Verification items for the finished model (mm, model axes). Face numbers are marked on the shaded views. A direction names the side the tool comes from. Give positions to 0.01 mm unless a question says otherwise; leave off trailing zeros. Loops run counter-clockwise (first coordinate to the right, second up) from the corner with the lowest first, then second, coordinate; pieces in that order, holes last. Notation, with made-up numbers: M -7.5,73.5 L 42.5,73.5 A25 ccw 42.5,89.5 Z; hole C 12.5,-35 d6. An arc over 180 degrees is marked long. Use CSV: the item, a comma, the result in double quotes.
from build123d import *

# Parameters (mm, degrees)
SKETCH1_W                 = 150
SKETCH1_H                 = 54.5
BOSS_EXTRUDE1_DEPTH       = 5
SKETCH2_W                 = 5
SKETCH2_H                 = 54.5
BOSS_EXTRUDE2_DEPTH       = 8
F_8_CLEARANCE_HOLE1_D     = 4.4958
F_8_CLEARANCE_HOLE1_DEPTH = 17
F_8_CLEARANCE_HOLE1_TIP   = 1.350674586
SKETCH7_W                 = 5
SKETCH7_H                 = 54.5
BOSS_EXTRUDE3_DEPTH       = 43
SKETCH8_R                 = 4.25
CUT_EXTRUDE1_DEPTH        = 4
RIB1_REACH                = 120.085
SKETCH10_WALL_W           = 279.571445908
SKETCH10_WALL_H           = 10
RIB3_REACH                = 120.085
SKETCH12_WALL_W           = 279.571445908
SKETCH12_WALL_H           = 10
SKETCH13_W                = 8
SKETCH13_H                = 2
BOSS_EXTRUDE4_DEPTH       = 5
SKETCH14_R                = 2
CUT_EXTRUDE2_DEPTH        = 2
SKETCH15_R                = 3.5
CUT_EXTRUDE3_DEPTH        = 1
F_8_CLEARANCE_HOLE2_D     = 4.4958
F_8_CLEARANCE_HOLE2_DEPTH = 17
F_8_CLEARANCE_HOLE2_TIP   = 1.350674586
SKETCH16_W                = 10
SKETCH16_H                = 12
BOSS_EXTRUDE5_DEPTH       = 20
SKETCH18_W                = 7
SKETCH18_H                = 7
CUT_EXTRUDE4_DEPTH        = 8


with BuildPart() as part:
    # Sketch1 → Boss-Extrude1 (new body)
    with BuildSketch(Plane(origin=(0, 0, 0), x_dir=(1, 0, 0), z_dir=(0, 1, 0))):
        with Locations((-18.112463826, -1.689393939)):
            Rectangle(SKETCH1_W, SKETCH1_H)
    extrude(amount=BOSS_EXTRUDE1_DEPTH)

    # Sketch2 → Boss-Extrude2 (add)
    with BuildSketch(Plane(origin=(0, 5, 0), x_dir=(1, 0, 0), z_dir=(0, 1, 0))):
        with Locations((-90.612463826, -1.689393939)):
            Rectangle(SKETCH2_W, SKETCH2_H)
    extrude(amount=BOSS_EXTRUDE2_DEPTH)

    # #8 Clearance Hole1
    with Locations(Plane(origin=(-93.112463826, 9.2, -15.560606061), x_dir=(0, 0, -1), z_dir=(-1, 0, 0))):
        with Locations((0, 0), (-17.25, 0), (-34.5, 0)):
            Hole(F_8_CLEARANCE_HOLE1_D / 2, depth=F_8_CLEARANCE_HOLE1_DEPTH)
            with Locations((0, 0, -(F_8_CLEARANCE_HOLE1_DEPTH + F_8_CLEARANCE_HOLE1_TIP / 2))):  # 118° drill point
                Cone(0, F_8_CLEARANCE_HOLE1_D / 2, F_8_CLEARANCE_HOLE1_TIP, mode=Mode.SUBTRACT)

    # Sketch7 → Boss-Extrude3 (add)
    with BuildSketch(Plane(origin=(0, 5, 0), x_dir=(1, 0, 0), z_dir=(0, 1, 0))):
        with Locations((54.387536174, -1.689393939)):
            Rectangle(SKETCH7_W, SKETCH7_H)
    extrude(amount=BOSS_EXTRUDE3_DEPTH)

    # Sketch8 → Cut-Extrude1 (cut)
    with BuildSketch(Plane.ZY.offset(-51.887536174)):
        with Locations((-15.560606061, 43)):
            Circle(SKETCH8_R)
        with Locations((18.939393939, 43)):
            Circle(SKETCH8_R)
    extrude(amount=-CUT_EXTRUDE1_DEPTH, mode=Mode.SUBTRACT)

    # Sketch10 wall → Rib1 (add, up to next)
    with BuildSketch(Plane(origin=(39.387536174, 21.5, -25.560606061), x_dir=(-0.603857687995, -0.797092148154, 0), z_dir=(-0.797092148154, 0.603857687995, 0)), mode=Mode.PRIVATE) as rib1_sk1:
        with Locations((0, 5)):
            Rectangle(SKETCH10_WALL_W, SKETCH10_WALL_H)
    rib1_tool1 = extrude(rib1_sk1.sketch, amount=-RIB1_REACH, mode=Mode.PRIVATE) - part.part
    add(rib1_tool1.solids().sort_by_distance((39.387536174, 21.5, -25.560606061))[0])

    # Sketch12 wall → Rib3 (add, up to next)
    with BuildSketch(Plane(origin=(39.387536174, 21.5, 28.939393939), x_dir=(-0.603857687995, -0.797092148154, 0), z_dir=(0.797092148154, -0.603857687995, 0)), mode=Mode.PRIVATE) as rib3_sk1:
        with Locations((0, 5)):
            Rectangle(SKETCH12_WALL_W, SKETCH12_WALL_H)
    rib3_tool1 = extrude(rib3_sk1.sketch, amount=RIB3_REACH, mode=Mode.PRIVATE) - part.part
    add(rib3_tool1.solids().sort_by_distance((39.387536174, 21.5, 28.939393939))[0])

    # Sketch13 → Boss-Extrude4 (add)
    with BuildSketch(Plane.ZY.offset(-51.887536174)):
        with Locations((1.689393939, 37)):
            Rectangle(SKETCH13_W, SKETCH13_H)
    extrude(amount=BOSS_EXTRUDE4_DEPTH)

    # Sketch14 → Cut-Extrude2 (cut)
    with BuildSketch(Plane(origin=(0, 38, 0), x_dir=(1, 0, 0), z_dir=(0, 1, 0))):
        with Locations(Location((49.387536174, -1.689393939, 0), (0, 0, 270))):
            Circle(SKETCH14_R)
    extrude(amount=-CUT_EXTRUDE2_DEPTH, mode=Mode.SUBTRACT)

    # Sketch15 → Cut-Extrude3 (cut)
    with BuildSketch(Plane.ZY.offset(-55.887536174)):
        with Locations((-15.560606061, 43)):
            Circle(SKETCH15_R)
        with Locations((18.939393939, 43)):
            Circle(SKETCH15_R)
    extrude(amount=-CUT_EXTRUDE3_DEPTH, mode=Mode.SUBTRACT)

    # #8 Clearance Hole2
    with Locations(Plane(origin=(-3.112463826, 5, 1.689393939), x_dir=(0, 0, 1), z_dir=(0, 1, 0))):
        with Locations((0, 0), (13.625, -30), (-13.625, -30)):
            Hole(F_8_CLEARANCE_HOLE2_D / 2, depth=F_8_CLEARANCE_HOLE2_DEPTH)
            with Locations((0, 0, -(F_8_CLEARANCE_HOLE2_DEPTH + F_8_CLEARANCE_HOLE2_TIP / 2))):  # 118° drill point
                Cone(0, F_8_CLEARANCE_HOLE2_D / 2, F_8_CLEARANCE_HOLE2_TIP, mode=Mode.SUBTRACT)

    # Sketch16 → Boss-Extrude5 (add)
    with BuildSketch(Plane(origin=(0, 5, 0), x_dir=(1, 0, 0), z_dir=(0, 1, 0))):
        with Locations((-6.112463826, 15.560606061)):
            Rectangle(SKETCH16_W, SKETCH16_H)
        with Locations((-6.112463826, -18.939393939)):
            Rectangle(SKETCH16_W, SKETCH16_H)
    extrude(amount=BOSS_EXTRUDE5_DEPTH)

    # Sketch18 → Cut-Extrude4 (cut)
    with BuildSketch(Plane.ZY.offset(11.112463826)):
        with Locations((-15.560606061, 20)):
            Rectangle(SKETCH18_W, SKETCH18_H)
        with Locations((18.939393939, 20)):
            Rectangle(SKETCH18_W, SKETCH18_H)
    extrude(amount=-CUT_EXTRUDE4_DEPTH, mode=Mode.SUBTRACT)


solid = part.part
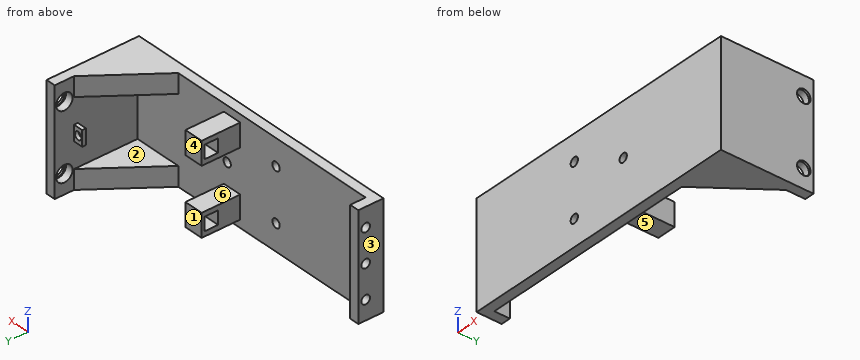
(1) Tool access check on the marked faces 4, 5 and 6. Record the directions out of +Z, -Z, +X, -X, +Y, -Y that give a thin tool (end or side, any length) a straight path to the whole face; none if there is none.
Calculated:
face 4,"+Z, -Z, -X, +Y"
face 5,"-Z, +Y"
face 6,"+Y"
(2) Scan lines: L1, parallel to Z at x = -90.7, y = 9.2; L2, parallel to Z at x = -89, y = 9; L3, parallel to X at y = 34, z = 18. Record each from-to range of solid material in increasing order. Write a range as from..to.
Calculated:
L1,"z = -25.56..-17.81, -13.31..-0.56, 3.94..16.69, 21.19..28.94"
L2,"z = -25.56..-17.8, -13.32..-0.55, 3.93..16.7, 21.18..28.94"
L3,"x = 51.89..56.89"
(3) Section check C-C on y = 9.2. Count the separate pieces of the cut face and the enclosed holes in it, plus the area to 3 significant figures.
Calculated:
separate pieces,"7"
enclosed holes,"0"
area,"1,150 mm²"
(4) Mould release check, pull along X, two halves, no side actions. Record for the marked faces 1, 2 and 3: released by +X, released by -X, zero draft, split by the parting line, or undercut.
Calculated:
face 1,"zero draft"
face 2,"undercut"
face 3,"released by -X"
(5) Section check A-A on x = -7.5. Record the cut outline in (y, z), plus the area to 4 significant figures.
Calculated:
outline,"M 0,-25.56 L 5,-25.56 L 5,-21.56 L 25,-21.56 L 25,-9.56 L 5,-9.56 L 5,12.94 L 25,12.94 L 25,24.94 L 5,24.94 L 5,28.94 L 0,28.94 Z; hole M 16.5,-19.06 L 23.5,-19.06 L 23.5,-12.06 L 16.5,-12.06 Z; hole M 16.5,15.44 L 23.5,15.44 L 23.5,22.44 L 16.5,22.44 Z"
area,"654.5 mm²"
(6) Section check B-B on y = 43. Record the cut outline in (x, z).
Calculated:
outline,"M 51.89,-25.56 L 56.89,-25.56 L 56.89,-19.06 L 55.89,-19.06 L 55.89,-19.81 L 51.89,-19.81 Z; M 51.89,-11.31 L 55.89,-11.31 L 55.89,-12.06 L 56.89,-12.06 L 56.89,15.44 L 55.89,15.44 L 55.89,14.69 L 51.89,14.69 Z; M 51.89,23.19 L 55.89,23.19 L 55.89,22.44 L 56.89,22.44 L 56.89,28.94 L 51.89,28.94 Z"
(7) Section check D-D on z = 9. Record the cut outline in (x, y), plus the area to 4 significant figures.
Calculated:
outline,"M -93.11,0 L 56.89,0 L 56.89,48 L 51.89,48 L 51.89,5 L -88.11,5 L -88.11,13 L -93.11,13 Z"
area,"1,005 mm²"
(8) Depth check by flat-ended pin: pin 1 Ø10 at (x, z) = (-10, -19.5) entering from +Y; pin 2 Ø5 at (x, z) = (-3.11, 1.69) entering from +Y; pin 3 Ø2.5 at (y, z) = (9.2, 18.94) entering from -X; pin 4 Ø5 at (y, z) = (43, -15.56) entering from -X. Enter the tip coordinate at first touch or a pass-through.
Calculated:
pin 1,"stops at y = 25"
pin 2,"stops at y = 5"
pin 3,"stops at x = -11.11"
pin 4,"passes through"
